Build history of the part. All positions in model axes, mm. Face numbers are marked on the shaded views. A direction names the side the tool comes from. Coordinates: 2 decimals unless noted, no trailing zeros. Write each loop counter-clockwise with the first axis right and the second up, starting at its lowest first coordinate (ties: lowest second). Pieces come first, ordered by that corner, then holes. Notation, with made-up numbers: (7.25, -32) -> (28.25, -32) arc R23 ccw to (28.25, -1) -> close; hole circle Ø11 at (-1.5, 36). An arc over 180 degrees is marked (long way). Write each question's results on one line, items separated by ' | '. Start each with the question number.
Q1. Drill centre lines: line 1 (Y direction, x = 2.5, z = 4); line 2 (Y direction, x = 1.25, z = 3.1); line 3 (X direction, y = 0.25, z = 4.25). Where is each one in solid material? Low to high.
Q2. Saw through at D-D on x = 3.25. Give the cut face in (y, z).
Q3. Two-plate mould, pull along X, no slides. Class the marked faces 1, 2 and 3: released by +X, released by -X, zero draft, split by the parting line, or undercut.
Q4. Saw through at C-C on z = 2.7. Count the separate pieces of the cut face and the enclosed holes in it, and give its area (3 significant figures).
Q5. Tool access for the marked faces 4 and 5: list every direction of +Z, -Z, +X, -X, +Y, -Y with a clear straight run to the whole face (end or side of a thin tool).
Q6. Saw through at B-B on z = 0.5. Give the cut face in (x, y).
Q7. Saw through at A-A on y = 0.85. Give the cut face in (x, z).
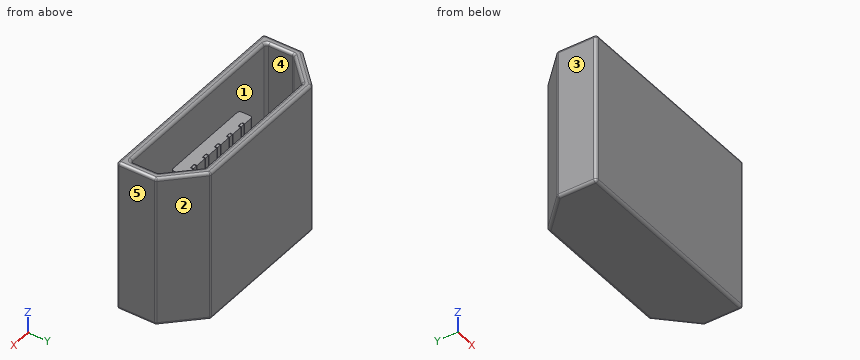
from build123d import *

# Parameters (mm, degrees)
EXTRUDE_THIN1_DEPTH = 5.5
BOSS_EXTRUDE1_DEPTH = 2.5
SKETCH3_W           = 3.5
SKETCH3_H           = 0.5
BOSS_EXTRUDE2_DEPTH = 1.65
SKETCH4_W           = 0.2
SKETCH4_H           = 0.1
CUT_EXTRUDE1_DEPTH  = 1.65
BOSS_EXTRUDE4_REACH = 6.15
SKETCH5_W           = 0.15
SKETCH5_H           = 0.09
FILLET1_R           = 0.1


with BuildPart() as part:
    # Sketch1 → Extrude-Thin1 (new body)
    with BuildSketch(Plane.XY):
        Polygon((-0.3, -0.3), (7.3, -0.3), (7.3, 1.124264069), (6.124264069, 2.3), (0.875735931, 2.3), (-0.3, 1.124264069), align=None)
        Polygon((0, 0), (7, 0), (7, 1), (6, 2), (1, 2), (0, 1), align=None, mode=Mode.SUBTRACT)
    extrude(amount=EXTRUDE_THIN1_DEPTH)

    # Sketch2 → Boss-Extrude1 (add)
    with BuildSketch(Plane(origin=(0, 0, 0), x_dir=(-1, 0, 0), z_dir=(0, 0, -1))):
        Polygon((-6, 2), (-1, 2), (0, 1), (0, 0), (-7, 0), (-7, 1), align=None)
    extrude(amount=-BOSS_EXTRUDE1_DEPTH)

    # Sketch3 → Boss-Extrude2 (add)
    with BuildSketch(Plane.XY.offset(2.5)):
        with Locations((3.5, 0.5)):
            Rectangle(SKETCH3_W, SKETCH3_H)
    extrude(amount=BOSS_EXTRUDE2_DEPTH)

    # Sketch4 → Cut-Extrude1 (cut)
    with BuildSketch(Plane.XY.offset(4.15)):
        with Locations((2.266666667, 0.7)):
            Rectangle(SKETCH4_W, SKETCH4_H)
        with Locations((2.883333333, 0.7)):
            Rectangle(SKETCH4_W, SKETCH4_H)
        with Locations((3.5, 0.7)):
            Rectangle(SKETCH4_W, SKETCH4_H)
        with Locations((4.116666667, 0.7)):
            Rectangle(SKETCH4_W, SKETCH4_H)
        with Locations((4.733333333, 0.7)):
            Rectangle(SKETCH4_W, SKETCH4_H)
    extrude(amount=-CUT_EXTRUDE1_DEPTH, mode=Mode.SUBTRACT)

    # Sketch5 → Boss-Extrude4 (add, up to next)
    with BuildSketch(Plane.XY.offset(4.15), mode=Mode.PRIVATE) as boss_extrude4_sk1:
        with Locations((2.266666667, 0.705)):
            Rectangle(SKETCH5_W, SKETCH5_H)
    boss_extrude4_tool1 = extrude(boss_extrude4_sk1.sketch, amount=-BOSS_EXTRUDE4_REACH, mode=Mode.PRIVATE) - part.part
    add(boss_extrude4_tool1.solids().sort_by_distance((2.266667, 0.705, 4.15))[0])
    # Sketch5 → Boss-Extrude4 (add, up to next)
    with BuildSketch(Plane.XY.offset(4.15), mode=Mode.PRIVATE) as boss_extrude4_sk2:
        with Locations((2.883333333, 0.705)):
            Rectangle(SKETCH5_W, SKETCH5_H)
    boss_extrude4_tool2 = extrude(boss_extrude4_sk2.sketch, amount=-BOSS_EXTRUDE4_REACH, mode=Mode.PRIVATE) - part.part
    add(boss_extrude4_tool2.solids().sort_by_distance((2.883333, 0.705, 4.15))[0])
    # Sketch5 → Boss-Extrude4 (add, up to next)
    with BuildSketch(Plane.XY.offset(4.15), mode=Mode.PRIVATE) as boss_extrude4_sk3:
        with Locations((3.5, 0.705)):
            Rectangle(SKETCH5_W, SKETCH5_H)
    boss_extrude4_tool3 = extrude(boss_extrude4_sk3.sketch, amount=-BOSS_EXTRUDE4_REACH, mode=Mode.PRIVATE) - part.part
    add(boss_extrude4_tool3.solids().sort_by_distance((3.5, 0.705, 4.15))[0])
    # Sketch5 → Boss-Extrude4 (add, up to next)
    with BuildSketch(Plane.XY.offset(4.15), mode=Mode.PRIVATE) as boss_extrude4_sk4:
        with Locations((4.116666667, 0.705)):
            Rectangle(SKETCH5_W, SKETCH5_H)
    boss_extrude4_tool4 = extrude(boss_extrude4_sk4.sketch, amount=-BOSS_EXTRUDE4_REACH, mode=Mode.PRIVATE) - part.part
    add(boss_extrude4_tool4.solids().sort_by_distance((4.116667, 0.705, 4.15))[0])
    # Sketch5 → Boss-Extrude4 (add, up to next)
    with BuildSketch(Plane.XY.offset(4.15), mode=Mode.PRIVATE) as boss_extrude4_sk5:
        with Locations((4.733333333, 0.705)):
            Rectangle(SKETCH5_W, SKETCH5_H)
    boss_extrude4_tool5 = extrude(boss_extrude4_sk5.sketch, amount=-BOSS_EXTRUDE4_REACH, mode=Mode.PRIVATE) - part.part
    add(boss_extrude4_tool5.solids().sort_by_distance((4.733333, 0.705, 4.15))[0])

    # Fillet1
    fillet1_edges = [part.edges().sort_by_distance(p)[0] for p in [
        (7.3, 0.412132034, 5.5),
        (6.712132034, 1.712132034, 5.5),
        (3.5, 2.3, 5.5),
        (0, 1, 4),
        (0.287867966, 1.712132034, 5.5),
        (0, 0, 4),
        (7, 0, 4),
        (7, 1, 4),
        (6, 2, 4),
        (1, 2, 4),
        (0, 0.5, 5.5),
        (3.5, 0, 5.5),
        (7, 0.5, 5.5),
        (6.5, 1.5, 5.5),
        (3.5, 2, 5.5),
        (0.5, 1.5, 5.5),
        (-0.3, 0.412132034, 5.5),
        (0.287867966, 1.712132034, 0),
        (3.5, 2.3, 0),
        (6.712132034, 1.712132034, 0),
        (7.3, 0.412132034, 0),
        (3.5, -0.3, 0),
        (-0.3, 0.412132034, 0),
        (1.75, 0.75, 3.325),
        (1.75, 0.25, 3.325),
        (5.25, 0.25, 3.325),
        (5.25, 0.75, 3.325),
        (3.5, -0.3, 5.5),
        (-0.3, 1.124264069, 2.75),
        (0.875735931, 2.3, 2.75),
        (6.124264069, 2.3, 2.75),
        (7.3, 1.124264069, 2.75),
        (7.3, -0.3, 2.75),
        (-0.3, -0.3, 2.75),
    ]]
    fillet(fillet1_edges, radius=FILLET1_R)


solid = part.part
Returned:
1) line 1: y = -0.3 to 0, 0.25 to 0.75, 2 to 2.3 | line 2: y = -0.3 to 0, 2 to 2.3 | line 3: x = -0.3 to 0, 7 to 7.3
2) outline: (-0.3, 0.1) arc R0.1 ccw to (-0.2, 0) -> (2.2, 0) arc R0.1 ccw to (2.3, 0.1) -> (2.3, 5.4) arc R0.1 ccw to (2.2, 5.5) -> (2.1, 5.5) arc R0.1 ccw to (2, 5.4) -> (2, 2.5) -> (0.75, 2.5) -> (0.75, 4.15) -> (0.25, 4.15) -> (0.25, 2.5) -> (0, 2.5) -> (0, 5.4) arc R0.1 ccw to (-0.1, 5.5) -> (-0.2, 5.5) arc R0.1 ccw to (-0.3, 5.4) -> close
3) face 1: undercut | face 2: released by +X | face 3: released by -X
4) separate pieces: 7 | enclosed holes: 1 | area: 7.09 mm2
5) face 4: +Z | face 5: +Z, -Z, +X, +Y, -Y
6) outline: (-0.3, -0.2) arc R0.1 ccw to (-0.2, -0.3) -> (7.2, -0.3) arc R0.1 ccw to (7.3, -0.2) -> (7.3, 1.08) arc R0.1 ccw to (7.27, 1.15) -> (6.15, 2.27) arc R0.1 ccw to (6.08, 2.3) -> (0.92, 2.3) arc R0.1 ccw to (0.85, 2.27) -> (-0.27, 1.15) arc R0.1 ccw to (-0.3, 1.08) -> close
7) outline: (-0.3, 0.1) arc R0.1 ccw to (-0.2, 0) -> (7.2, 0) arc R0.1 ccw to (7.3, 0.1) -> (7.3, 5.4) arc R0.1 ccw to (7.2, 5.5) -> (7.1, 5.5) arc R0.1 ccw to (7, 5.4) -> (7, 2.5) -> (0, 2.5) -> (0, 5.4) arc R0.1 ccw to (-0.1, 5.5) -> (-0.2, 5.5) arc R0.1 ccw to (-0.3, 5.4) -> close
